from build123d import *

# Parameters (mm, degrees)
EXTRUDE_1_DEPTH      = 26
SKETCH_4_R           = 9.996910884
CUT_EXTRUDE_2_DEPTH  = 26
FILLET_1_R           = 10
FILLET_2_R           = 10
CUT_EXTRUDE_4_DEPTH  = 26
SKETCH_8_R           = 13.6
CUT_EXTRUDE_5_DEPTH  = 20.12
EXTRUDE_2_DEPTH      = 26
FILLET_3_R           = 3
CUT_EXTRUDE_6_DEPTH  = 30
FILLET_9_R           = 10
FILLET_10_R          = 3
FILLET_11_R          = 10
CUT_EXTRUDE_7_DEPTH  = 30
SKETCH_13_W          = 20.118493956
SKETCH_13_H          = 70
CUT_EXTRUDE_8_DEPTH  = 44.75
CUT_EXTRUDE_9_DEPTH  = 44.75
SKETCH_15_R          = 22
EXTRUDE_3_DEPTH      = 26
EXTRUDE_4_REACH      = 99.657
CUT_EXTRUDE_13_DEPTH = 20
EXTRUDE_START        = -2.941506044
EXTRUDE_5_DEPTH      = 2.941506044
EXTRUDE_6_DEPTH      = 2.94


with BuildPart() as part:
    # 草图1 → 凸台-拉伸1 (new body)
    with BuildSketch(Plane.XY):
        Polygon((0, 0), (60.004097951, 0), (60.004097951, 25.002996284), (-59.998288516, 25.002996284), (-59.998288516, 0), align=None)
    extrude(amount=EXTRUDE_1_DEPTH)

    # 草图4 → 切除-拉伸2 (cut)
    with BuildSketch(Plane.XY.offset(26)):
        with Locations((-47.497668288, 12.501498142)):
            Circle(SKETCH_4_R)
    extrude(amount=-CUT_EXTRUDE_2_DEPTH, mode=Mode.SUBTRACT)

    # 圆角1
    fillet_1_edges = [part.edges().sort_by_distance(p)[0] for p in [
        (-59.998288516, 25.002996284, 13),
    ]]
    fillet(fillet_1_edges, radius=FILLET_1_R)

    # 圆角2
    fillet_2_edges = [part.edges().sort_by_distance(p)[0] for p in [
        (-59.998288516, 0, 13),
    ]]
    fillet(fillet_2_edges, radius=FILLET_2_R)

    # 草图7 → 切除-拉伸4 (cut)
    with BuildSketch(Plane(origin=(0, 25.002996284, 0), x_dir=(1, 0, 0), z_dir=(0, 1, 0))):
        Polygon((-37.501471928, -23.058493956), (-36.401101967, -23.058493956), (-36.401101967, -2.94), (-37.501471928, -2.94), (-62.053584156, -2.94), (-62.053584156, -23.058493956), align=None)
    extrude(amount=-CUT_EXTRUDE_4_DEPTH, mode=Mode.SUBTRACT)

    # 草图8 → 切除-拉伸5 (cut)
    with BuildSketch(Plane.XY.offset(2.94)):
        with Locations((-47.497668288, 12.501498142)):
            Circle(SKETCH_8_R)
    extrude(amount=CUT_EXTRUDE_5_DEPTH, mode=Mode.SUBTRACT)

    # 草图9 → 凸台-拉伸2 (add)
    with BuildSketch(Plane.XY.offset(26)):
        Polygon((-34.9988745, 25.002996284), (-22.500080712, 12.501498142), (-27.68722448, 0), (39.366276038, -67.053500518), (48.202948014, -58.216828542), (57.0397416, -49.380034956), (-17.34328964, 25.002996284), (-26.17108207, 33.830788714), align=None)
    extrude(amount=-EXTRUDE_2_DEPTH)

    # 圆角3
    fillet_3_edges = [part.edges().sort_by_distance(p)[0] for p in [
        (-36.401101967, 0, 12.999246978),
        (-36.401101967, 20.36446297, 12.999246978),
        (-36.401101967, 4.638533314, 12.999246978),
    ]]
    fillet(fillet_3_edges, radius=FILLET_3_R)

    # 草图10 → 切除-拉伸6 (cut)
    with BuildSketch(Plane.XY.offset(26)):
        Polygon((7.659706645, 0), (60.004097951, 0), (60.004097951, 25.002996284), (-17.34328964, 25.002996284), align=None)
    extrude(amount=-CUT_EXTRUDE_6_DEPTH, mode=Mode.SUBTRACT)

    # 圆角9
    # the kernel refuses this fillet: 10 mm, written as the material it adds along each edge
    with BuildSketch(Plane(origin=(-34.9988745, 25.002996284, 26), x_dir=(-1, 0, 0), z_dir=(0, 0, -1))) as fillet_9_piece_1_section:
        with BuildLine():
            CenterArc((FILLET_9_R * 0.414213562373, FILLET_9_R), FILLET_9_R, 225, 45)
            Line((-FILLET_9_R * 0.292893218813, FILLET_9_R * 0.292893218813), (0, 0))
            Line((0, 0), (FILLET_9_R * 0.414213562373, 0))
        make_face()
    fillet_9_piece_1 = extrude(amount=26, mode=Mode.PRIVATE)
    fillet_9_piece_1 = split(fillet_9_piece_1, bisect_by=Plane(origin=(-36.401101967, 24.986097048, 24.529246978), z_dir=(-1, 0, 0)), keep=Keep.TOP, mode=Mode.PRIVATE)
    fillet_9_piece_1 = split(fillet_9_piece_1, bisect_by=Plane(origin=(-37.504554949, 24.986097048, 23.058493956), z_dir=(0, 0, 1)), keep=Keep.TOP, mode=Mode.PRIVATE)
    add(fillet_9_piece_1)
    with BuildSketch(Plane(origin=(-34.9988745, 25.002996284, 26), x_dir=(-1, 0, 0), z_dir=(0, 0, -1))) as fillet_9_piece_2_section:
        with BuildLine():
            CenterArc((FILLET_9_R * 0.414213562373, FILLET_9_R), FILLET_9_R, 225, 45)
            Line((-FILLET_9_R * 0.292893218813, FILLET_9_R * 0.292893218813), (0, 0))
            Line((0, 0), (FILLET_9_R * 0.414213562373, 0))
        make_face()
    fillet_9_piece_2 = extrude(amount=26, mode=Mode.PRIVATE)
    fillet_9_piece_2 = split(fillet_9_piece_2, bisect_by=Plane(origin=(-36.401101967, 25.815006688, 24.529246978), z_dir=(1, 0, 0)), keep=Keep.TOP, mode=Mode.PRIVATE)
    fillet_9_piece_2 = split(fillet_9_piece_2, bisect_by=Plane(origin=(-34.567927652, 25.815006688, 23.058493956), z_dir=(0, 0, 1)), keep=Keep.TOP, mode=Mode.PRIVATE)
    add(fillet_9_piece_2)
    with BuildSketch(Plane(origin=(-34.9988745, 25.002996284, 26), x_dir=(-1, 0, 0), z_dir=(0, 0, -1))) as fillet_9_piece_3_section:
        with BuildLine():
            CenterArc((FILLET_9_R * 0.414213562373, FILLET_9_R), FILLET_9_R, 225, 45)
            Line((-FILLET_9_R * 0.292893218813, FILLET_9_R * 0.292893218813), (0, 0))
            Line((0, 0), (FILLET_9_R * 0.414213562373, 0))
        make_face()
    fillet_9_piece_3 = extrude(amount=26, mode=Mode.PRIVATE)
    fillet_9_piece_3 = split(fillet_9_piece_3, bisect_by=Plane(origin=(-34.567927652, 25.815006688, 2.94), z_dir=(0, 0, 1)), keep=Keep.TOP, mode=Mode.PRIVATE)
    fillet_9_piece_3 = split(fillet_9_piece_3, bisect_by=Plane(origin=(-36.401101967, 25.815006688, 12.999246978), z_dir=(1, 0, 0)), keep=Keep.TOP, mode=Mode.PRIVATE)
    fillet_9_piece_3 = split(fillet_9_piece_3, bisect_by=Plane(origin=(-34.567927652, 25.815006688, 23.058493956), z_dir=(0, 0, -1)), keep=Keep.TOP, mode=Mode.PRIVATE)
    add(fillet_9_piece_3)
    with BuildSketch(Plane(origin=(-34.9988745, 25.002996284, 26), x_dir=(-1, 0, 0), z_dir=(0, 0, -1))) as fillet_9_piece_4_section:
        with BuildLine():
            CenterArc((FILLET_9_R * 0.414213562373, FILLET_9_R), FILLET_9_R, 225, 45)
            Line((-FILLET_9_R * 0.292893218813, FILLET_9_R * 0.292893218813), (0, 0))
            Line((0, 0), (FILLET_9_R * 0.414213562373, 0))
        make_face()
    fillet_9_piece_4 = extrude(amount=26, mode=Mode.PRIVATE)
    fillet_9_piece_4 = split(fillet_9_piece_4, bisect_by=Plane(origin=(-37.504554949, 24.986097048, 2.94), z_dir=(0, 0, -1)), keep=Keep.TOP, mode=Mode.PRIVATE)
    fillet_9_piece_4 = split(fillet_9_piece_4, bisect_by=Plane(origin=(-36.401101967, 24.986097048, 1.47), z_dir=(-1, 0, 0)), keep=Keep.TOP, mode=Mode.PRIVATE)
    add(fillet_9_piece_4)
    with BuildSketch(Plane(origin=(-34.9988745, 25.002996284, 26), x_dir=(-1, 0, 0), z_dir=(0, 0, -1))) as fillet_9_piece_5_section:
        with BuildLine():
            CenterArc((FILLET_9_R * 0.414213562373, FILLET_9_R), FILLET_9_R, 225, 45)
            Line((-FILLET_9_R * 0.292893218813, FILLET_9_R * 0.292893218813), (0, 0))
            Line((0, 0), (FILLET_9_R * 0.414213562373, 0))
        make_face()
    fillet_9_piece_5 = extrude(amount=26, mode=Mode.PRIVATE)
    fillet_9_piece_5 = split(fillet_9_piece_5, bisect_by=Plane(origin=(-34.567927652, 25.815006688, 2.94), z_dir=(0, 0, -1)), keep=Keep.TOP, mode=Mode.PRIVATE)
    fillet_9_piece_5 = split(fillet_9_piece_5, bisect_by=Plane(origin=(-36.401101967, 25.815006688, 1.47), z_dir=(1, 0, 0)), keep=Keep.TOP, mode=Mode.PRIVATE)
    add(fillet_9_piece_5)

    # 圆角10
    fillet_10_edges = [part.edges().sort_by_distance(p)[0] for p in [
        (-36.401101967, 25.385673201, 12.999246978),
    ]]
    fillet(fillet_10_edges, radius=FILLET_10_R)

    # 圆角11
    fillet_11_edges = [part.edges().sort_by_distance(p)[0] for p in [
        (-26.17108207, 33.830788714, 13),
    ]]
    fillet(fillet_11_edges, radius=FILLET_11_R)

    # 草图12 → 切除-拉伸7 (cut)
    with BuildSketch(Plane(origin=(3.829853322, 3.829853322, 0), x_dir=(0, 0, -1), z_dir=(0.7071067811865404, 0.7071067811865547, 0))):
        Polygon((-12.999246978, 43.121170069), (-9.998089183, 43.121170069), (-9.998089183, 23.118852005), (-15.995491838, 23.118852005), (-15.995491838, 43.121170069), align=None)
    extrude(amount=-CUT_EXTRUDE_7_DEPTH, mode=Mode.SUBTRACT)

    # 草图13 → 切除-拉伸8 (cut, symmetric)
    with BuildSketch(Plane(origin=(3.829853322, 3.829853322, 0), x_dir=(0, 0, -1), z_dir=(0.7071067811865404, 0.7071067811865547, 0))):
        with Locations((-12.999246978, 7.961145372)):
            Rectangle(SKETCH_13_W, SKETCH_13_H)
    extrude(amount=CUT_EXTRUDE_8_DEPTH, both=True, mode=Mode.SUBTRACT)

    # 草图14 → 切除-拉伸9 (cut, symmetric)
    with BuildSketch(Plane(origin=(3.829853322, 3.829853322, 0), x_dir=(0, 0, -1), z_dir=(0.7071067811865404, 0.7071067811865547, 0))):
        Polygon((-23.06, 55.962849268), (-23.058493956, 36.05981453), (-2.94, 36.05981453), (-2.94, 55.962849268), align=None)
    extrude(amount=CUT_EXTRUDE_9_DEPTH, both=True, mode=Mode.SUBTRACT)

    # 草图15 → 凸台-拉伸3 (add)
    with BuildSketch(Plane(origin=(0, 0, 0), x_dir=(-1, 0, 0), z_dir=(0, 0, -1))):
        with Locations((-39.366276038, -49.380034956)):
            Circle(SKETCH_15_R)
    extrude(amount=-EXTRUDE_3_DEPTH)

    # 凸台-拉伸4: up to this face of the body (flat: up to its plane)
    extrude_4_end = Plane(part.part.faces().sort_by_distance((10.252727371, -21.880412524, 0))[0])
    # 草图16 → 凸台-拉伸4 (add, up to the picked face)
    with BuildSketch(Plane.XY.offset(26), mode=Mode.PRIVATE) as extrude_4_sk1:
        with BuildLine():
            Line((53.281607925, -32.339978076), (-19.148678719, 26.808385364))
            Line((-19.148678719, 26.808385364), (35.400190623, -27.740483979))
            ThreePointArc((35.400190623, -27.740483979), (44.846760764, -28.073597263), (53.281607925, -32.339978076))
        make_face()
    extrude_4_tool1 = split(extrude(extrude_4_sk1.sketch, amount=-EXTRUDE_4_REACH, mode=Mode.PRIVATE), bisect_by=extrude_4_end, keep=Keep.BOTH, mode=Mode.PRIVATE)
    add(extrude_4_tool1.solids().sort_by(Axis((21.577836, -9.730931, 26), (0, 0, -1)))[0])

    # 草图17 → 切除-拉伸13 (cut)
    with BuildSketch(Plane(origin=(3.829853322, 3.829853322, 0), x_dir=(0, 0, 1), z_dir=(-0.7071067811865404, -0.7071067811865548, 0))):
        Polygon((23.058493956, 32.496551656), (23.058493956, -27.038854628), (2.94, -27.038854628), (2.94, 32.428906565), (2.94, 35.354128857), (23.06, 35.354128857), align=None)
    extrude(amount=-CUT_EXTRUDE_13_DEPTH, mode=Mode.SUBTRACT)

    # 草图19 → 凸台-拉伸5 (add)
    with BuildSketch(Plane.XY.offset(26).offset(EXTRUDE_START)):
        with BuildLine():
            Line((-32.763505202, 0), (-27.68722448, 0))
            Line((-27.68722448, 0), (17.726725061, -45.413949541))
            ThreePointArc((17.726725061, -45.413949541), (17.874446419, -54.081232636), (21.358890569, -62.018629363))
            Line((21.358890569, -62.018629363), (-32.763505202, 0))
        make_face()
    extrude(amount=EXTRUDE_5_DEPTH)

    # 草图20 → 凸台-拉伸6 (add)
    with BuildSketch(Plane(origin=(0, 0, 0), x_dir=(-1, 0, 0), z_dir=(0, 0, -1))):
        with BuildLine():
            Line((-17.726725061, -45.413949541), (27.68722448, 0))
            Line((27.68722448, 0), (32.763505202, 0))
            Line((32.763505202, 0), (-21.358890569, -62.018629363))
            ThreePointArc((-21.358890569, -62.018629363), (-17.874446419, -54.081232636), (-17.726725061, -45.413949541))
        make_face()
    extrude(amount=-EXTRUDE_6_DEPTH)


solid = part.part
Work out the finished part from the listing and answer in its coordinate system (mm). A direction names the side the tool comes from. Round coordinates to 2 decimals unless told otherwise and drop trailing zeros. Write each loop counter-clockwise with the first axis right and the second up, starting at its lowest first coordinate (ties: lowest second). Pieces come first, ordered by that corner, then holes. Notation, with made-up numbers: (-20, 85) -> (-13, 85) arc R24 cw to (-13, 100) -> close; hole circle Ø3 at (-12, 47). An arc over 180 degrees is marked (long way). Answer as CSV lines item,"result". Start each with the question number.
(1) A tool of negligible diameter and unlimited length cuts with its end or side. For faces 4 (the flat face through (-41, 21, 23.06)), 5 (the flat face through (-44, 25.003, 25)), 6 (the flat face through (-5.323, -31.443, 24.509)), from which of +Z, -Z, +X, -X, +Y, -Y can it reach the whole face along a straight path? Write none if from no direction.
(2) Each of these flat-tipped pins is pushed along its axis until it touches: pin 1 (3 mm diameter, centred on y = -52.5, z = 8.5, fed in from -X); pin 2 (0.9 mm diameter, centred on x = -43, z = 24, fed in from +Y); pin 3 (5 mm diameter, centred on y = -1.5, z = 22.5, fed in from +X). Where does it stop, or does it pass through?
(3) The part is cut by section D-D, the plane x = 13.5. Give the vertices of the cut face in (y, z).
(4) The mould has two halves that part along Z. Classify faces 1 (the flat face through (16.084, -22.155, 13.14)), 2 (the flat face through (13, -20, 0)), 3 (the flat face through (-42, 0, 25)): +Z half, -Z half, draft (parallel to the pull), parting line (faces both ways), or undercut.
(5) The part is cut by section A-A, the plane x = -52. Give the vertices of the cut face in (y, z).
(6) Find the intervals of material crossed by probe 1 along Z at (x, y) = (-35.5, 17); probe 2 along Y at (x, z) = (-43, 1.75); probe 3 along X at (y, z) = (-31, 11), in increasing order.
(7) The part is cut by section B-B, the plane y = -22. Give the vertices of the cut face in (x, z).
(8) The part is cut by section C-C, the plane z = 14.25. Give the vertices of the cut face in (x, y).
Output values:
1,face 4,"+X, -X, +Y, -Y"
1,face 5,"+Z, -Z, -X, +Y"
1,face 6,"+Z, -Z, -X, -Y"
2,pin 1,"stops at x = 17.43"
2,pin 2,"stops at y = 25"
2,pin 3,"stops at x = 18.5"
3,outline,"(-53.01, 0) -> (0.15, 0) -> (0.15, 2.94) -> (-24.74, 2.94) -> (-24.74, 23.06) -> (0.15, 23.06) -> (0.15, 26) -> (-53.01, 26) -> (-53.01, 23.06) -> (-41.19, 23.06) -> (-41.19, 2.94) -> (-53.01, 2.94) -> close"
4,face 1,"undercut"
4,face 2,"-Z half"
4,face 3,"draft"
5,outline,"(0.2, 0) -> (3.58, 0) -> (3.58, 2.94) -> (0.2, 2.94) -> close; (0.2, 23.06) -> (3.58, 23.06) -> (3.58, 26) -> (0.2, 26) -> close; (21.43, 0) -> (24.8, 0) -> (24.8, 2.94) -> (21.43, 2.94) -> close; (21.43, 23.06) -> (24.8, 23.06) -> (24.8, 26) -> (21.43, 26) -> close"
6,probe 1,"z = 0 to 2.94, 23.06 to 26"
6,probe 2,"y = 0 to 3.57, 21.43 to 25"
6,probe 3,"x = 7.24 to 51.64"
7,outline,"(-13.56, 0) -> (40.62, 0) -> (40.62, 26) -> (-13.56, 26) -> (-13.56, 23.06) -> (16.24, 23.06) -> (16.24, 2.94) -> (-13.56, 2.94) -> close"
8,outline,"(5.28, -32.96) -> (17.73, -45.41) arc R22 ccw (long way) to (53.28, -32.34) -> (27.2, -11.04) -> close"
